```python
from build123d import *

# Parameters (mm, degrees)
SKETCH_W     = 45
SKETCH_H     = 45
PAD_DEPTH    = 78
POCKET_DEPTH = 45.001


with BuildPart() as part:
    # Sketch → Pad (new body)
    with BuildSketch(Plane.XY):
        with Locations((-22.5, 22.5)):
            Rectangle(SKETCH_W, SKETCH_H)
    extrude(amount=PAD_DEPTH)

    # Sketch001 (on Face1 of Pad) → Pocket (cut, through all)
    with BuildSketch(Plane.XZ):
        Polygon((-12, 0), (0, 72), (0, 0), align=None)
    extrude(amount=-POCKET_DEPTH, mode=Mode.SUBTRACT)


solid = part.part
```
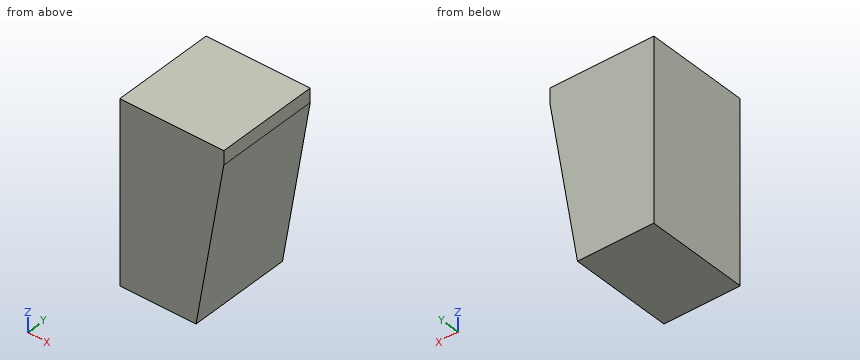
Can you work these out from the model? Positions are in its coordinate system, mm. Give positions to 0.01 mm unless a question says otherwise; leave off trailing zeros. Loops run counter-clockwise (first coordinate to the right, second up) from the corner with the lowest first, then second, coordinate; pieces in that order, holes last. Notation, with made-up numbers: M 39,21 L 96,21 A30 cw 96,48 Z; hole C -7.5,82 d2. An arc over 180 degrees is marked long. One line per item, written item: value.
(1) I need wall thicknesses on line 1 (X direction, y = 11, z = 46.5); line 2 (X direction, y = 13.5, z = 37.5). Which ranges of each line are inside material? Lowest first, please.
Returned:
line 1: -45 to -4.25
line 2: -45 to -5.75
(2) Suppose I cut it at B-B on x = -10.5. List the corners of the cut face in (y, z) for me, plus the area to 4 significant figures.
Returned:
outline: M 0,9 L 45,9 L 45,78 L 0,78 Z
area: 3,105 mm^2
(3) Suppose I cut it at A-A on y = 11.5. List the corners of the cut face in (x, z) for me, plus the area to 3 significant figures.
Returned:
outline: M -45,0 L -12,0 L 0,72 L 0,78 L -45,78 Z
area: 3,080 mm^2
(4) Suppose I cut it at C-C on z = 40. List the corners of the cut face in (x, y) for me.
Returned:
outline: M -45,0 L -5.33,0 L -5.33,45 L -45,45 Z
(5) Will these pins go through, and if not, where does the flat tip stop? pin 1 (5 mm diameter, centred on y = 9.5, z = 68, fed in from +X); pin 2 (6 mm diameter, centred on x = -23.5, z = 44.5, fed in from -Y); pin 3 (10 mm diameter, centred on y = 5.5, z = 11.5, fed in from +X).
Returned:
pin 1: x = -0.25
pin 2: y = 0
pin 3: x = -9.25
